Autodesk Inventor part; units mm, degrees
ref_plane "YZ Plane" through (0, 0, 0) normal (1, 0, 0) x (0, 1, 0)
ref_plane "XZ Plane" through (0, 0, 0) normal (0, 1, 0) x (-1, 0, 0)
ref_plane "XY Plane" through (0, 0, 0) normal (0, 0, 1) x (1, 0, 0)
sketch "Sketch1" plane through (0, 0, 0) normal (0, 1, 0) x (-1, 0, 0)
  line L0 (-13.5, 16) -> (-10.5, 16)
  line L1 (-22.2016, 21.0925) -> (-25.0207, 22.1185)
  line L2 (-10.5, 31) -> (-13.5, 31)
  line L3 (-10.5, 16) -> (-10.5, 31)
  line L4 (-19.8904, 36.2139) -> (-17.0713, 35.1879)
  line L5 (-13.5, 45) -> (-17.0713, 35.1879)
  line L6 (-13.5, 45) -> (-13.5, 31)
  line L7 (-13.5, -14) -> (-32.4622, -7.0983)
  line L8 (-27.3319, 6.9971) -> (-22.2016, 21.0925)
  line L9 (-22.2016, 21.0925) -> (-27.3319, 6.9971)
  line L10 (-13.5, 1) -> (-13.5, 16)
  line L11 (-13.5, 16) -> (-13.5, 1)
  line L12 (-30.151, 8.0231) -> (-27.3319, 6.9971)
  line L13 (-10.5, 1) -> (-13.5, 1)
  line L14 (-13.5, -14) -> (-10.5, -14)
  line L15 (-10.5, -14) -> (-10.5, 1)
  line L16 (-32.4622, -7.0983) -> (-35.2813, -6.0723)
  line L17 (-27.3319, 6.9971) -> (-32.0304, 8.7072)
  line L18 (-32.0304, 8.7072) -> (-37.1607, -5.3882)
  line L19 (-37.1607, -5.3882) -> (-35.2813, -6.0723)
  line L20 (-25.0207, 22.1185) -> (-26.9001, 22.8026)
  line L21 (-26.9001, 22.8026) -> (-21.7698, 36.898)
  line L22 (-21.7698, 36.898) -> (-19.8904, 36.2139)
  point P0 (0, 0)
  point P1 (0, 0)
  dimension "d0" = 3
  dimension "d1" = 15
  dimension "d2" = 15
  dimension "d3" = 15
  dimension "d4" = 15
  dimension "d5" = 15
  dimension "d6" = 15
  dimension "d7" = 2.8191
  dimension "d8" = 5
extrude "Extrusion1" add sketch "Sketch1" along normal blind 3
properties part number "do_sensor_3_3mm"
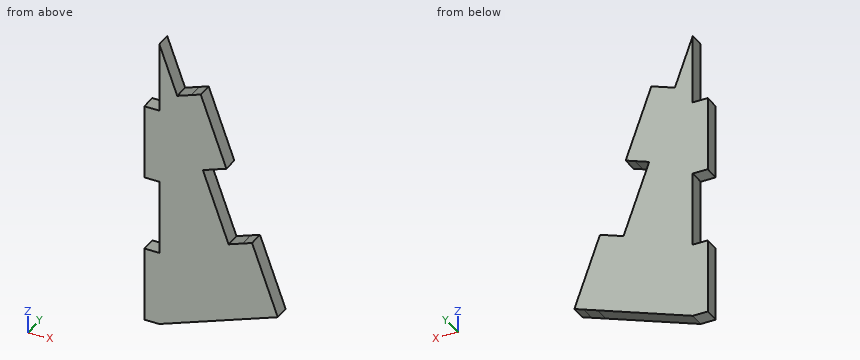
Design review of the part built by this model. Coordinates are the model's own, in mm. Coordinates: 2 decimals unless noted, no trailing zeros. Loops run counter-clockwise (first coordinate to the right, second up) from the corner with the lowest first, then second, coordinate; pieces in that order, holes last. Notation, with made-up numbers: (52, 30.5) -> (101, 30.5) arc R16 cw to (101, 56.5) -> close; hole circle Ø6 at (66.5, 75.5). An arc over 180 degrees is marked (long way). Answer as a JSON object with one key per item and string values.
Q1. Take a section at B-B on z = 3. Give the boundary of the cut face in (x, y).
Answer block:
{"outline": "(13.5, 0) -> (34.11, 0) -> (34.11, 3) -> (13.5, 3) -> close"}
Q2. To check wall thickness, follow L1, parallel to Z at x = 12.75, y = 2.8; L2, parallel to X at y = 0.7, z = 14; L3, parallel to X at y = 1.15, z = 12.5. State the ranges of each line that lie inside material, in increasing order.
Answer block:
{"L1": "z = -14 to 1, 16 to 31", "L2": "x = 13.5 to 24.78", "L3": "x = 13.5 to 25.33"}
Q3. Clearance check with a flat-ended pin moving along its axis: pin 1 Ø0.9 at (x, y) = (11.5, 1.5) entering from +Z. State where the tip first meets the part, or that it passes through.
Answer block:
{"pin 1": "stops at z = 31"}
Q4. Take a section at C-C on x = 20.5. Give the boundary of the cut face in (y, z).
Answer block:
{"outline": "(0, -11.45) -> (3, -11.45) -> (3, 36.44) -> (0, 36.44) -> close"}
Q5. Take a section at A-A on y = 1.2. Give the boundary of the cut face in (x, z), plus the area to 3 significant figures.
Answer block:
{"outline": "(10.5, -14) -> (13.5, -14) -> (32.46, -7.1) -> (35.28, -6.07) -> (37.16, -5.39) -> (32.03, 8.71) -> (30.15, 8.02) -> (27.33, 7) -> (22.2, 21.09) -> (25.02, 22.12) -> (26.9, 22.8) -> (21.77, 36.9) -> (19.89, 36.21) -> (17.07, 35.19) -> (13.5, 45) -> (13.5, 31) -> (10.5, 31) -> (10.5, 16) -> (13.5, 16) -> (13.5, 1) -> (10.5, 1) -> close", "area": "799 mm^2"}
